from build123d import *

# Parameters (mm, degrees)
SKETCH1_R                = 2.6
BOSS_EXTRUDE1_DEPTH      = 7
SKETCH3_R                = 20
CUT_EXTRUDE1_DEPTH       = 105.322688225
BOSS_EXTRUDE2_DEPTH      = 75
BOSS_EXTRUDE3_DEPTH      = 10
BOSS_EXTRUDE3_DEPTH_BACK = 20
SKETCH5_R                = 28.5


with BuildPart() as part:
    # Sketch1 → Boss-Extrude1 (new body)
    with BuildSketch(Plane.XY):
        Polygon((-81.297129584, 62), (-81.297129584, 25.5), (-81.297129584, 8), (-78.297129584, 8), (-41.797129584, 8), (-24.297129584, 8), (-24.297129584, 11), (-24.297129584, 47.5), (-24.297129584, 65), (-27.297129584, 65), (-63.797129584, 65), (-81.297129584, 65), align=None)
        with Locations((-76.297129584, 13)):
            Circle(SKETCH1_R, mode=Mode.SUBTRACT)
        with Locations((-29.297129584, 13)):
            Circle(SKETCH1_R, mode=Mode.SUBTRACT)
        with Locations((-29.297129584, 60)):
            Circle(SKETCH1_R, mode=Mode.SUBTRACT)
        with Locations((-76.297129584, 60)):
            Circle(SKETCH1_R, mode=Mode.SUBTRACT)
    extrude(amount=BOSS_EXTRUDE1_DEPTH)

    # Sketch3 → Cut-Extrude1 (cut, through all)
    with BuildSketch(Plane.XY.offset(7)):
        with Locations((-52.797129584, 36.5)):
            Circle(SKETCH3_R)
    extrude(amount=-CUT_EXTRUDE1_DEPTH, mode=Mode.SUBTRACT)

    # Sketch4 → Boss-Extrude2 (add)
    with BuildSketch(Plane.XY.offset(7)):
        Polygon((-24.297129584, 65), (-17.297129584, 65), (-17.297129584, 1), (-88.297129584, 1), (-88.297129584, 65), (-81.297129584, 65), (-81.297129584, 8), (-24.297129584, 8), align=None)
    extrude(amount=-BOSS_EXTRUDE2_DEPTH)

    # Sketch5 → Boss-Extrude3 (add, two sides: drawn at the far end of the back side and taken through both)
    with BuildSketch(Plane(origin=(0, 0, -68), x_dir=(-1, 0, 0), z_dir=(0, 0, -1)).offset(-BOSS_EXTRUDE3_DEPTH_BACK)):
        Polygon((88.297129584, 1), (88.297129584, -74), (52.797129584, -74), (17.297129584, -74), (17.297129584, 1), (17.297129584, 65), (24.297129584, 65), (24.297129584, 8), (81.297129584, 8), (81.297129584, 65), (88.297129584, 65), align=None)
        with Locations((52.797129584, -36.5)):
            Circle(SKETCH5_R, mode=Mode.SUBTRACT)
    extrude(amount=BOSS_EXTRUDE3_DEPTH + BOSS_EXTRUDE3_DEPTH_BACK)


solid = part.part
Check sheet for the modelled part. Datum: model origin and axes. Units: mm. A direction names the side the tool comes from. Give positions to 0.01 mm unless a question says otherwise; leave off trailing zeros. Write each loop counter-clockwise with the first axis right and the second up, starting at its lowest first coordinate (ties: lowest second). Pieces come first, ordered by that corner, then holes. Notation, with made-up numbers: (53, -36) -> (99, -36) arc R26 ccw to (99, -15) -> close; hole circle Ø11 at (36, 79). An arc over 180 degrees is marked (long way). Write item = value, one per line.
Item 1: Sectioned sample at B-B on z = -54. Record the boundary of the cut face in (x, y).
Output:
outline = (-88.3, -74) -> (-17.3, -74) -> (-17.3, 65) -> (-24.3, 65) -> (-24.3, 8) -> (-81.3, 8) -> (-81.3, 65) -> (-88.3, 65) -> close; hole circle Ø57 at (-52.8, -36.5)
Item 2: Gauge pin test, flat ends, axial feed: pin 1 (17 mm diameter, centred on x = -48, z = -48.5, fed in from +Y); pin 2 (6 mm diameter, centred on x = -73.5, z = -28.5, fed in from -Y); pin 3 (7 mm diameter, centred on x = -76.3, y = 13, fed in from +Z). Record the tip position at first contact, or that the pin passes through.
Output:
pin_1 = 8
pin_2 = 1
pin_3 = 7
Item 3: Release check for a two-part mould opening along Y. For faces 4 (the cylindrical face through (-67.538, 50.017, 3.549)), 5 (the flat face through (-17.297, 12, -44)), 6 (the flat face through (-24, 65, -26)) record: +Y half, -Y half, draft (parallel to the pull), parting line (faces both ways), or undercut.
Output:
face_4 = undercut
face_5 = draft
face_6 = +Y half
Item 4: Sectioned sample at D-D on y = 60. Record the boundary of the cut face in (x, z).
Output:
outline = (-88.3, -78) -> (-81.3, -78) -> (-81.3, 0) -> (-78.9, 0) -> (-78.9, 7) -> (-88.3, 7) -> close; (-73.7, 0) -> (-31.9, 0) -> (-31.9, 7) -> (-73.7, 7) -> close; (-26.7, 0) -> (-24.3, 0) -> (-24.3, -78) -> (-17.3, -78) -> (-17.3, 7) -> (-26.7, 7) -> close
Item 5: Sectioned sample at C-C on x = -55.5. Record the boundary of the cut face in (y, z).
Output:
outline = (-74, -78) -> (-64.87, -78) -> (-64.87, -48) -> (-74, -48) -> close; (-8.13, -78) -> (8, -78) -> (8, 0) -> (16.68, 0) -> (16.68, 7) -> (1, 7) -> (1, -48) -> (-8.13, -48) -> close; (56.32, 0) -> (65, 0) -> (65, 7) -> (56.32, 7) -> close
Item 6: Scan lines: probe 1 along X at (y, z) = (38.5, -47); probe 2 along Y at (x, z) = (-31.5, -37.5); probe 3 along Z at (x, y) = (-26.5, 22). Record each from-to range of solid material in increasing order. Write a range as from..to.
Output:
probe_1 = -88.3..-81.3, -24.3..-17.3
probe_2 = 1..8
probe_3 = 0..7
Item 7: Sectioned sample at A-A on y = 36.5. Record the boundary of the cut face in (x, z).
Output:
outline = (-88.3, -78) -> (-81.3, -78) -> (-81.3, 0) -> (-72.8, 0) -> (-72.8, 7) -> (-88.3, 7) -> close; (-32.8, 0) -> (-24.3, 0) -> (-24.3, -78) -> (-17.3, -78) -> (-17.3, 7) -> (-32.8, 7) -> close
Item 8: Tool access check on faces 1 (the flat face through (-60, 56, 0)), 2 (the flat face through (-52, 1, -20)), 3 (the cylindrical face through (-31.36, 11.42, 3.45)). Record the directions out of +Z, -Z, +X, -X, +Y, -Y that give a thin tool (end or side, any length) a straight path to the whole face; none if there is none.
Output:
face_1 = -Z, +Y
face_2 = +Z, +X, -X, -Y
face_3 = +Z, -Z
